The model under review builds one solid part; all positions refer to its coordinate system, in mm. Face numbers are marked on the shaded views. Coordinates: 2 decimals unless noted, no trailing zeros. Loops run counter-clockwise (first coordinate to the right, second up) from the corner with the lowest first, then second, coordinate; pieces in that order, holes last. Notation, with made-up numbers: (71.5, -19.5) - (88.5, -19.5) arc R22 ccw to (88.5, 11.5) - close; hole circle Ø2 at (62.25, 31.25). An arc over 180 degrees is marked (long way). Answer in a Markdown table with one row per item. Add a question column.
(1) We need section C-C on z = 2.5. Write out the cut boundary in (x, y) (1 decimal).
(2) We need section B-B on x = 35.5. Write out the cut boundary in (y, z) (3 decimals).
(3) We need section A-A on y = 4.5. Write out the cut boundary in (x, z).
(4) For P1, Ø1, axis at x = 36, y = 13.5, coming from the -Z side, flat-tipped, find the tip position at first contact; note if it passes through.
(5) Mouldability with a two-part tool opening along Z and no side actions: class the marked faces 1 and 2 as +Z half, -Z half, draft (parallel to the pull), parting line (faces both ways), or undercut.
(6) For line 1 along Y through (x, z) = (38, 2.25) (1 decimal); line 2 along Y through (x, z) = (19, 2.45) (1 decimal); line 3 along X through (y, z) = (7, 2.1), list the stretches that pass through material, from the lowest coordinate up.
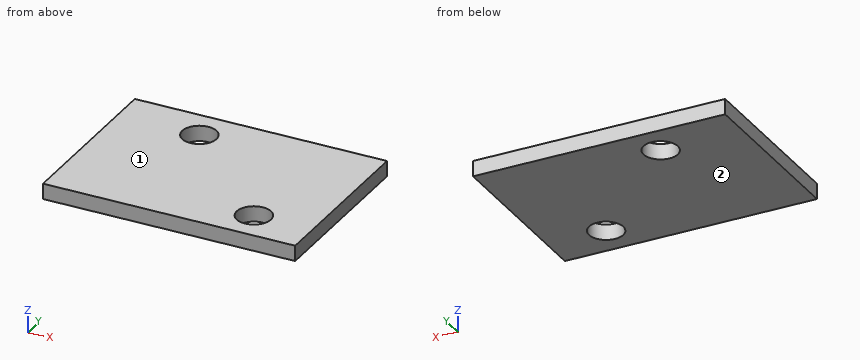
Autodesk Inventor part; units mm, degrees
ref_plane "YZ Plane" through (0, 0, 0) normal (1, 0, 0) x (0, 1, 0)
ref_plane "XZ Plane" through (0, 0, 0) normal (0, 1, 0) x (-1, 0, 0)
ref_plane "XY Plane" through (0, 0, 0) normal (0, 0, 1) x (1, 0, 0)
sketch "Sketch1" plane through (0, 0, 0) normal (0, 0, 1) x (1, 0, 0)
  line L0 (0, 0) -> (49.53, 0)
  line L1 (49.53, 0) -> (49.53, 34.925)
  line L2 (49.53, 34.925) -> (0, 34.925)
  line L3 (0, 34.925) -> (0, 0)
  dimension "d0" = 49.53
  dimension "d1" = 34.925
extrude "Plate1" add sketch "Sketch1" along normal blind 3.048
hole "Hole1" at (38.0365, 6.5532, 3.048) direction (0, 0, -1) diameter 6.731 end through all
hole "Hole2" at (16.0528, 28.3845, 3.048) direction (0, 0, -1) diameter 6.731 end through all
equation "\"d10\" = Thickness"
equation "\"d20\" = Thickness"
equation "\"BendRadius\" = Thickness"
equation "\"BendReliefWidth\" = Thickness"
equation "\"BendReliefDepth\" = 0.5 * Thickness"
equation "\"CornerReliefSize\" = 4 * Thickness"
equation "\"MinimumRemnant\" = 2 * Thickness"
equation "\"TransitionRadius\" = BendRadius"
equation "\"JacobiRadiusSize\" = BendRadius"
equation "\"GapSize\" = Thickness"
equation "\"d2\" = BendRadius"
properties part number "Claw - Arm - Plate 2"
Outcome:
| question | item | result |
|---|---|---|
| 1 | outline | (0, 0) - (49.5, 0) - (49.5, 34.9) - (0, 34.9) - close; hole circle Ø6.7 at (16.1, 28.4); hole circle Ø6.7 at (38, 6.6) |
| 2 | outline | (0, 0) - (4.341, 0) - (4.341, 3.048) - (0, 3.048) - close; (8.765, 0) - (34.925, 0) - (34.925, 3.048) - (8.765, 3.048) - close |
| 3 | outline | (0, 0) - (35.37, 0) - (35.37, 3.05) - (0, 3.05) - close; (40.7, 0) - (49.53, 0) - (49.53, 3.05) - (40.7, 3.05) - close |
| 4 | P1 | z = 0 |
| 5 | face 1 | +Z half |
| 5 | face 2 | -Z half |
| 6 | line 1 | 0 to 3.2, 9.9 to 34.9 |
| 6 | line 2 | 0 to 26.8, 30 to 34.9 |
| 6 | line 3 | 0 to 34.7, 41.37 to 49.53 |
